Input: part model. Units: mm. Frame: model coordinates. A direction names the side the tool comes from. Give positions to 0.01 mm unless a question says otherwise; leave off trailing zeros. Loops run counter-clockwise (first coordinate to the right, second up) from the corner with the lowest first, then second, coordinate; pieces in that order, holes last. Notation, with made-up numbers: M -14,61.5 L -10,61.5 A7 ccw -10,65.5 Z; hole C -40,16.5 d1. An arc over 180 degrees is marked long. Answer as a JSON object with one key per item and string values. Group by question number.
```python
from build123d import *

# Parameters (mm, degrees)
BASE_FLANGE1_DEPTH            = 3
EDGE_FLANGE2_STRIP_W          = 13.4732
EDGE_FLANGE2_STRIP_H          = 3
EDGE_FLANGE2_STRIP_CUT_DEPTH  = 349.93
EDGE_FLANGE2_RELIEF_W         = 14.9732
EDGE_FLANGE2_RELIEF_H         = 1.5
EDGE_FLANGE2_RELIEF_CUT_DEPTH = 3
EDGE_FLANGE2_DEPTH            = 349.93
CUT_EXTRUDE1_DEPTH            = 372.023186472
CUT_EXTRUDE1_DEPTH_BACK       = 372.023186472
SKETCH22_R                    = 4.075
SKETCH22_R_2                  = 11.075
SKETCH22_R_3                  = 1.575
CUT_EXTRUDE2_DEPTH            = 372.023186472
CUT_EXTRUDE2_DEPTH_BACK       = 372.023186472
FILLET1_R                     = 2
CUT_EXTRUDE3_DEPTH            = 372.023186472
CUT_EXTRUDE3_DEPTH_BACK       = 372.023186472
SKETCH24_W                    = 100
SKETCH24_H                    = 5.2366
FILLET2_R                     = 1.5


# Sheet-metal steps are written as plain solids
with BuildPart() as part:
    # Sketch1 → Base-Flange1 (new body)
    with BuildSketch(Plane.XY):
        with BuildLine():
            Line((0, 13), (349.93, 13))
            ThreePointArc((349.93, 13), (366.054515497, -18.832159566), (330.851215972, -13))
            Line((330.851215972, -13), (0, -13))
            ThreePointArc((0, -13), (-13, 0), (0, 13))
        make_face()
    extrude(amount=-BASE_FLANGE1_DEPTH)

    # Edge-Flange2 strip (across the edge) → Edge-Flange2 strip cut (cut)
    with BuildSketch(Plane(origin=(349.93, 13, 0), x_dir=(0, -1, 0), z_dir=(-1, 0, 0))):
        with Locations((-6, -1.5)):
            Rectangle(EDGE_FLANGE2_STRIP_W, EDGE_FLANGE2_STRIP_H)
    extrude(amount=EDGE_FLANGE2_STRIP_CUT_DEPTH, mode=Mode.SUBTRACT)

    # Edge-Flange2 relief (on the sheet) → Edge-Flange2 relief cut (cut)
    with BuildSketch(Plane(origin=(349.93, 12.2634, 0), x_dir=(0, -1, 0), z_dir=(0, 0, 1))):
        with Locations((-5.9866, 0.75)):
            Rectangle(EDGE_FLANGE2_RELIEF_W, EDGE_FLANGE2_RELIEF_H)
        with Locations((-5.9866, -350.68)):
            Rectangle(EDGE_FLANGE2_RELIEF_W, EDGE_FLANGE2_RELIEF_H)
    extrude(amount=-EDGE_FLANGE2_RELIEF_CUT_DEPTH, mode=Mode.SUBTRACT)

    # Edge-Flange2 section (across the edge) → Edge-Flange2 (add)
    with BuildSketch(Plane(origin=(349.93, 13, 0), x_dir=(0, -1, 0), z_dir=(-1, 0, 0))):
        with BuildLine():
            Line((-3, 0.7366), (-3, 9))
            Line((-3, 9), (0, 9))
            Line((0, 9), (0, 0.7366))
            ThreePointArc((0, 0.7366), (0.215745145, 0.215745145), (0.7366, 0))
            Line((0.7366, 0), (0.7366, -3))
            ThreePointArc((0.7366, -3), (-1.905575199, -1.905575199), (-3, 0.7366))
        make_face()
    extrude(amount=EDGE_FLANGE2_DEPTH)

    # Sketch22 → Cut-Extrude1 (cut, two sides: drawn at the far end of the back side and taken through both)
    with BuildSketch(Plane.XY.offset(-CUT_EXTRUDE1_DEPTH_BACK)):
        Circle(SKETCH22_R)
        with Locations((349.93, -7)):
            Circle(SKETCH22_R_2)
        with Locations((364.93, -7)):
            Circle(SKETCH22_R_3)
        with Locations((342.43, 5.990381057)):
            Circle(SKETCH22_R_3)
        with Locations((342.43, -19.990381057)):
            Circle(SKETCH22_R_3)
    extrude(amount=CUT_EXTRUDE1_DEPTH + CUT_EXTRUDE1_DEPTH_BACK, mode=Mode.SUBTRACT)

    # Sketch23 → Cut-Extrude2 (cut, two sides: drawn at the far end of the back side and taken through both)
    with BuildSketch(Plane.XY.offset(-CUT_EXTRUDE2_DEPTH_BACK)):
        Polygon((12.5, 6.5), (12.5, -6.5), (111.651399385, -6.5), align=None)
        Polygon((327.5, -6.5), (327.5, 6.5), (227.5, 6.5), align=None)
        Polygon((50.961538462, 6.5), (163.478075869, -8.252338296), (180.961538462, 6.5), align=None)
        Polygon((173.308112114, -6.5), (288.714823182, -6.5), (188.714823182, 6.5), align=None)
    extrude(amount=CUT_EXTRUDE2_DEPTH + CUT_EXTRUDE2_DEPTH_BACK, mode=Mode.SUBTRACT)

    # Fillet1
    fillet1_edges = [part.edges().sort_by_distance(p)[0] for p in [
        (327.5, -6.5, -1.5),
        (227.5, 6.5, -1.5),
        (327.5, 6.5, -1.5),
        (50.961538462, 6.5, -1.5),
        (180.961538462, 6.5, -1.5),
        (163.478075869, -8.252338296, -1.5),
        (173.308112114, -6.5, -1.5),
        (188.714823182, 6.5, -1.5),
        (288.714823182, -6.5, -1.5),
        (12.5, 6.5, -1.5),
        (111.651399385, -6.5, -1.5),
        (12.5, -6.5, -1.5),
        (349.93, 14.5, 9),
        (0, 14.5, 9),
    ]]
    fillet(fillet1_edges, radius=FILLET1_R)

    # Sketch24 → Cut-Extrude3 (cut, two sides: drawn at the far end of the back side and taken through both)
    with BuildSketch(Plane.XY.offset(-CUT_EXTRUDE3_DEPTH_BACK)):
        with Locations((50, 13.3817)):
            Rectangle(SKETCH24_W, SKETCH24_H)
        with Locations((299.93, 13.3817)):
            Rectangle(SKETCH24_W, SKETCH24_H)
    extrude(amount=CUT_EXTRUDE3_DEPTH + CUT_EXTRUDE3_DEPTH_BACK, mode=Mode.SUBTRACT)

    # Fillet2
    fillet2_edges = [part.edges().sort_by_distance(p)[0] for p in [
        (351.43, 12.943670675, -1.5),
        (-1.5, 12.91317157, -1.5),
        (100, 14.5, 9),
        (249.93, 14.5, 9),
    ]]
    fillet(fillet2_edges, radius=FILLET2_R)


solid = part.part
```
1. Section B-B (z = 4). Output: boundary loops of the cut face in (x, y).
2. Material intervals for L1, parallel to Y at x = 342.43, z = -0.9; L2, parallel to Z at x = 333, y = -9; L3, parallel to Y at x = 162, z = 7.25, sorted ascending.
3. Mould query, pull axis Y, two halves, no side actions, for faces 1 (the cylindrical face through (-3.234, -2.48, -1.521)), 2 (the flat face through (181, -7, 0)), 3 (the cylindrical face through (365.42, -19.65, -1.48)), 4 (the flat face through (176, 13, 5)). Classes: pulls with the +Y half, pulls with the -Y half, needs draft (parallel to the pull), parting line crosses it, or undercut.
4. Section A-A (x = 26). Output: boundary loops of the cut face in (y, z).
5. First-contact query: P1, Ø10, axis at x = 50, y = 8, coming from the +Z side; P2, Ø2.5, axis at x = 218.5, z = -2, coming from the -Y side; P3, Ø0.9, axis at y = -1, z = -2, coming from the -X side; P4, Ø3, axis at x = 364.93, y = -7, coming from the -Z side. Flat tips, straight axial feed; report the tip coordinate or a pass-through.
6. Reachability of faces 5 (the flat face through (182.839, 1.542, -1.521)), 6 (the flat face through (181, -7, -3)) from +Z, -Z, +X, -X, +Y, -Y: full face, straight path, thin tool, end or side. Return the list, or none.
Geometry results:
{
 "1": {"outline": "M 100,13 L 249.93,13 L 249.93,16 L 100,16 Z"},
 "2": {"L1": "-25.54 to -21.57, -18.42 to -15.15, 1.15 to 4.42, 7.57 to 10.76", "L2": "-3 to 0", "L3": "13 to 16"},
 "3": {"face 1": "undercut", "face 2": "needs draft", "face 3": "parting line crosses it", "face 4": "pulls with the -Y half"},
 "4": {"outline": "M -13,-3 L -6.5,-3 L -6.5,0 L -13,0 Z; M 4.73,-3 L 10.76,-3 L 10.76,0 L 4.73,0 Z"},
 "5": {"P1": "z = 0", "P2": "y = -13", "P3": "x = -12.99", "P4": "through"},
 "6": {"face 5": "+Z, -Z", "face 6": "-Z, +X, -X, +Y, -Y"}
}
